```python
from build123d import *

# Parameters (mm, degrees)
F0_R     = 117.5
F1_DEPTH = 220
F1_TAPER = -4
F2_T     = -5
F3_D     = 5
F3_DEPTH = 200
F3_TIP   = 1.5021515476


with BuildPart() as f1:
    # F0 (on Front) → F1 (new body)
    with BuildSketch(Plane.XZ):
        Circle(F0_R)
    extrude(amount=F1_DEPTH, taper=F1_TAPER)

    # F2
    f2_openings = [f1.faces().sort_by_distance(p)[0] for p in [
        (0, -220, 0),
    ]]
    offset(amount=F2_T, openings=f2_openings, kind=Kind.INTERSECTION)

    # F3
    with Locations(Plane(origin=(0, 0, 0), x_dir=(1, 0, 0), z_dir=(0, 1, 0))):
        with Locations((9.2098470777, -6.3473079354), (-8.0020800233, 7.90218357), (9.2098470777, 7.90218357), (0.3570861008, 32.7808782458), (18.7991485, 18.2122346014), (28.6735072732, 0), (18.7991485, -16.3738597184), (0.3570861008, -30.838817358), (-16.0174295306, -13.5970693082), (-28.4521393478, -24.2303218693), (-33.0149792135, 0), (-19.9558455497, 18.2122346014), (28.6735072732, 32.7808782458), (43.748550117, 20.8710134029), (53.2127507031, 0), (43.748550117, -21.4388202876), (28.6735072732, -28.6175906658), (28.6735072732, -48.8199926913), (0.3570861008, -56.4701706171), (-22.1440792084, -53.3896423876), (-46.6648377478, -43.2039052248), (-50.3848642111, -21.4388202876), (-54.3274022639, -3.6370723974), (-46.6648377478, 21.4596614242), (-33.0149792135, 32.7808782458), (-11.2309148535, 48.322789371), (18.7991485, 51.032319665), (-46.6648377478, 51.032319665), (-56.4857274294, 60.8595944941), (-69.0967813134, 72.2940042615), (43.748550117, 41.3127802312), (70.3815743327, 30.1224850118), (75.1331150532, 0), (70.3650861979, -34.0410172939), (43.748550117, -43.2039052248), (53.2127507031, -53.3896423876), (38.2187478244, -74.4572579861), (0.3570861008, -74.4572579861), (-35.8369350433, -74.4572579861), (-66.4791688323, -62.4554567039), (-74.753895402, -40.3432734311), (-74.753895402, -3.6370723974), (-74.753895402, 29.8503562808), (-33.0149792135, 72.2940042615), (-46.6648377478, 91.0002738237), (-17.2949098051, 96.9403386116), (0, 72.2940042615), (18.7991485, 96.9403386116), (38.2187478244, 72.2940042615), (53.2127507031, 93.0623114109), (75.8273825049, 71.850605309), (63.6254251003, 60.8595944941), (53.2127507031, 51.032319665), (88.8997167349, 51.032319665), (98.1507152319, 18.2122346014), (96.4434146881, -15.8068593591), (88.8997167349, -43.2039052248), (75.6580084562, -78.9676755667), (63.6254251003, -66.5364265442), (43.748550117, -92.5594046712), (22.1365932375, -100.0308543444), (-8.0020800233, -101.5365570784), (-41.1964207888, -92.5594046712), (-78.2781466842, -74.4572579861), (-96.2497368455, -43.2039052248), (-102.3866385221, -6.3473079354), (-96.2497368455, 27.1397344768)):
            Hole(F3_D / 2, depth=F3_DEPTH)
            with Locations((0, 0, -(F3_DEPTH + F3_TIP / 2))):  # 118° drill point
                Cone(0, F3_D / 2, F3_TIP, mode=Mode.SUBTRACT)


solid = f1.part
```
Read the model definition and answer for the solid it produces. Units are mm, in the model's axes. Give positions to 0.01 mm unless a question says otherwise; leave off trailing zeros. Order: outer loops, then holes, each group sorted by start corner. A loop starts at its lowest first (then second) coordinate and runs counter-clockwise, first axis right, second up. Notation, with made-up numbers: (7, 22) -> (63, 22) arc R29 cw to (63, 57) -> close; hole circle Ø8 at (-7, -15.75). An arc over 180 degrees is marked (long way). Write item = value, one per line.
1. The mould has two halves that part along Z. Classify faces 1 (the face through (-70, -220, 109)), 2 (the face through (-27.16, -111.54, -122.32)), 3 (the face through (-2, -5, 2)), 4 (the face through (-95.59, -114, -73.3)): +Z half, -Z half, draft (parallel to the pull), parting line (faces both ways), or undercut.
Numbers:
face_1 = draft
face_2 = parting line
face_3 = undercut
face_4 = undercut
2. Straight lines are drawn through the part: line 1 along Z through (x, y) = (0, -2.95); line 2 along X through (y, z) = (-201.5, 18); line 3 along Y through (x, z) = (5, -81.5). For each, find the intervals that lie inside material, in ascending order.
Numbers:
line_1 = -117.71 to -74.79, -69.79 to -35.26, -30.31 to 28.36, 33.31 to 54, 58.94 to 71.98, 76.93 to 117.71
line_2 = -130.35 to -125.29, 125.29 to 130.35
line_3 = -5 to 0
3. A cutting plane is placed at A-A, the plane y = -136. Write down the section's boundary in (x, z), and give its area (3 significant figures).
Numbers:
outline = circle Ø254.02 at (0, 0); hole circle Ø244 at (0, 0)
area = 3,920 mm²
4. Given pin 1 (6 mm diameter, centred on x = 38.22, z = 74.46, fed in from -Y); pin 2 (4 mm diameter, centred on x = 46.5, y = -146.5, fed in from +Z); pin 3 (6 mm diameter, centred on x = -56.49, z = -60.86, fed in from +Y); pin 4 (2 mm diameter, centred on y = -40.5, z = -66.5, fed in from -X), each flat-ended and moving along its own axis, determine where each tip first touches the part or whether it passes through.
Numbers:
pin_1 = -5
pin_2 = 119.76
pin_3 = 0
pin_4 = -100.95
5. A cutting plane is placed at B-B, the plane y = -33.5. Write down the section's boundary in (x, z), and give its area (3 significant figures).
Numbers:
outline = circle Ø239.69 at (0, 0); hole circle Ø229.66 at (0, 0)
area = 3,700 mm²
